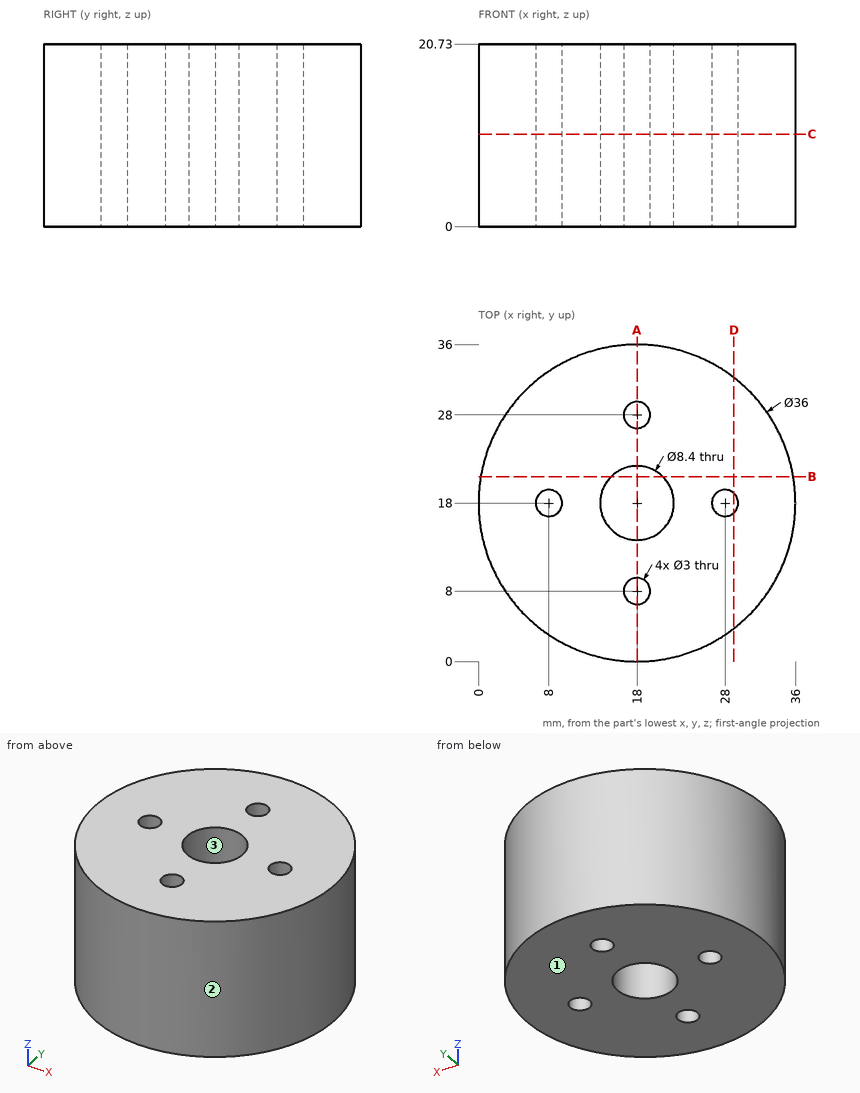
Design review of the part shown in the three views and the two pictorial views. Dimensions are in mm from the part's minimum x, y and z. Give positions to 0.01 mm unless a question says otherwise; leave off trailing zeros. Write each loop counter-clockwise with the first axis right and the second up, starting at its lowest first coordinate (ties: lowest second). Pieces come first, ordered by that corner, then holes. Notation, with made-up numbers: M 46.25,0 L 85.25,0 A10 ccw 85.25,8 Z; hole C 80,18 d11. An arc over 180 degrees is marked long. One line per question, with ' | ' between items. Start each with the question number.
Item 1: We need section B-B on y = 21. Write out the cut boundary in (x, z), plus the area to 3 significant figures.
Item 2: For pin 1 (12 mm diameter, centred on x = 25.5, z = 13.5, fed in from +Y); pin 2 (4 mm diameter, centred on y = 10, z = 7, fed in from -X); pin 3 (1 mm diameter, centred on x = 5.5, z = 10, fed in from +Y); pin 4 (2.5 mm diameter, centred on x = 28, y = 18, fed in from +Z), all flat-tipped, find the tip position at first contact; note any pin that passes through.
Item 3: We need section C-C on z = 10.5. Write out the cut boundary in (x, y), plus the area to 3 significant figures.
Item 4: We need section D-D on x = 29. Write out the cut boundary in (y, z), plus the area to 3 significant figures.
Item 5: Wall thickness on line 1 (Y direction, x = 18, z = 6); line 2 (Y direction, x = 15, z = 17); line 3 (X direction, y = 27.5, z = 9): over which ranges is each line inside the solid? List them lowest first. Write a range as from..to.
Item 6: Draft analysis for pull direction X (two halves, no side actions). For the marked faces 1, 2 and 3, state which applies: released by +X, released by -X, zero draft, split by the parting line, or undercut.
Item 7: We need section A-A on x = 18. Write out the cut boundary in (y, z).
Results found:
1) outline: M 0.25,0 L 15.06,0 L 15.06,20.73 L 0.25,20.73 Z; M 20.94,0 L 35.75,0 L 35.75,20.73 L 20.94,20.73 Z | area: 614 mm2
2) pin 1: stops at y = 35.94 | pin 2: stops at x = 1.03 | pin 3: stops at y = 31.42 | pin 4: passes through
3) outline: C 18,18 d36; hole C 8,18 d3; hole C 18,18 d8.4; hole C 18,8 d3; hole C 18,28 d3; hole C 28,18 d3 | area: 934 mm2
4) outline: M 3.75,0 L 16.88,0 L 16.88,20.73 L 3.75,20.73 Z; M 19.12,0 L 32.25,0 L 32.25,20.73 L 19.12,20.73 Z | area: 544 mm2
5) line 1: y = 0..6.5, 9.5..13.8, 22.2..26.5, 29.5..36 | line 2: y = 0.25..15.06, 20.94..35.75 | line 3: x = 2.71..16.59, 19.41..33.29
6) face 1: zero draft | face 2: split by the parting line | face 3: undercut
7) outline: M 0,0 L 6.5,0 L 6.5,20.73 L 0,20.73 Z; M 9.5,0 L 13.8,0 L 13.8,20.73 L 9.5,20.73 Z; M 22.2,0 L 26.5,0 L 26.5,20.73 L 22.2,20.73 Z; M 29.5,0 L 36,0 L 36,20.73 L 29.5,20.73 Z
